CAD build for the part. Positions are in the model's coordinates, mm. Face numbers are marked on the shaded views. Give positions to 0.01 mm unless a question says otherwise; leave off trailing zeros. Order: outer loops, then holes, each group sorted by start corner. A loop starts at its lowest first (then second) coordinate and runs counter-clockwise, first axis right, second up.
Autodesk Inventor part; units mm, degrees
ref_plane "YZ Plane" through (0, 0, 0) normal (1, 0, 0) x (0, 1, 0)
ref_plane "XZ Plane" through (0, 0, 0) normal (0, 1, 0) x (-1, 0, 0)
ref_plane "XY Plane" through (0, 0, 0) normal (0, 0, 1) x (1, 0, 0)
sketch "スケッチ1" plane through (0, 0, 0) normal (0, 0, 1) x (1, 0, 0)
  circle A0 centre (0, 0) radius 4
  circle A1 centre (0, 0) radius 2
  dimension "d0" = 8
  dimension "d1" = 4
extrude "押し出し1" add sketch "スケッチ1" along normal blind 45 contours A0 | A1
sketch "スケッチ2" plane through (0, 0, 45) normal (0, 0, 1) x (1, 0, 0)
  circle A0 centre (0, 0) radius 2
  dimension "d4" = 4
extrude "押し出し2" cut sketch "スケッチ2" against normal blind 8
sketch "スケッチ3" plane through (0, 0, 0) normal (0, 0, -1) x (-1, 0, 0)
  circle A0 centre (0, 0) radius 2
  dimension "d7" = 4
extrude "押し出し3" cut sketch "スケッチ3" against normal blind 8
properties part number "スペーサーm4,45" material "アルミニウム 7075"
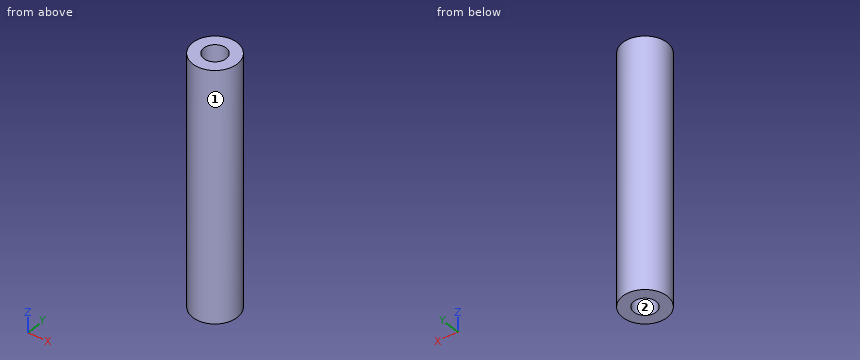
1. Saw through at B-B on z = 41. Give the cut face in (x, y).
2. Pin check, flat tips, straight feed: P1, Ø2, axis at x = 1.5, z = 5, coming from the -Y side; P2, Ø2, axis at x = 0.5, y = 0, coming from the +Z side. Stop position of each tip, or through.
3. Mould opens along X. For the marked faces 1 and 2 say: released by +X, released by -X, zero draft, split by the parting line, or undercut.
4. Wall check: line 1 (Y direction, x = 0, z = 39.5); line 2 (Z direction, x = -0.25, y = 1); line 3 (X direction, y = 1.5, z = 38). Give the ranges that are in metal, low to high.
5. Saw through at C-C on x = -1.25. Give the cut face in (y, z).
6. Saw through at D-D on z = 19. Give the cut face in (x, y), plus the area to 3 significant figures.
7. Saw through at A-A on y = 0. Give the cut face in (x, z).
Reported:
1. outline: circle Ø8 at (0, 0); hole circle Ø4 at (0, 0)
2. P1: stops at y = -3.97
2. P2: stops at z = 37
3. face 1: split by the parting line
3. face 2: undercut
4. line 1: y = -4 to -2, 2 to 4
4. line 2: z = 8 to 37
4. line 3: x = -3.71 to -1.32, 1.32 to 3.71
5. outline: (-3.8, 0) - (-1.56, 0) - (-1.56, 8) - (1.56, 8) - (1.56, 0) - (3.8, 0) - (3.8, 45) - (1.56, 45) - (1.56, 37) - (-1.56, 37) - (-1.56, 45) - (-3.8, 45) - close
6. outline: circle Ø8 at (0, 0)
6. area: 50.3 mm2
7. outline: (-4, 0) - (-2, 0) - (-2, 8) - (2, 8) - (2, 0) - (4, 0) - (4, 45) - (2, 45) - (2, 37) - (-2, 37) - (-2, 45) - (-4, 45) - close
